Job drawing, mm, ordinate dimensions from the low corner. One solid piece. Round coordinates to 2 decimals unless told otherwise and drop trailing zeros. Write each loop counter-clockwise with the first axis right and the second up, starting at its lowest first coordinate (ties: lowest second). Pieces come first, ordered by that corner, then holes.
1) Saw through at A-A (z = 58). Write the cut outline in (x, y).
2) Saw through at C-C (x = 2.3). Write the cut outline in (y, z), plus the area to 3 significant figures.
3) Saw through at B-B (y = 88). Write the cut outline in (x, z).
4) Saw through at D-D (z = 7.5). Write the cut outline in (x, y).
5) Wall check: probe 1 along Y at (x, z) = (2.7, 7.5); probe 2 along Z at (x, y) = (3.35, 105); probe 3 along Y at (x, z) = (2, 58). Give the ranges that are in metal, low to high.
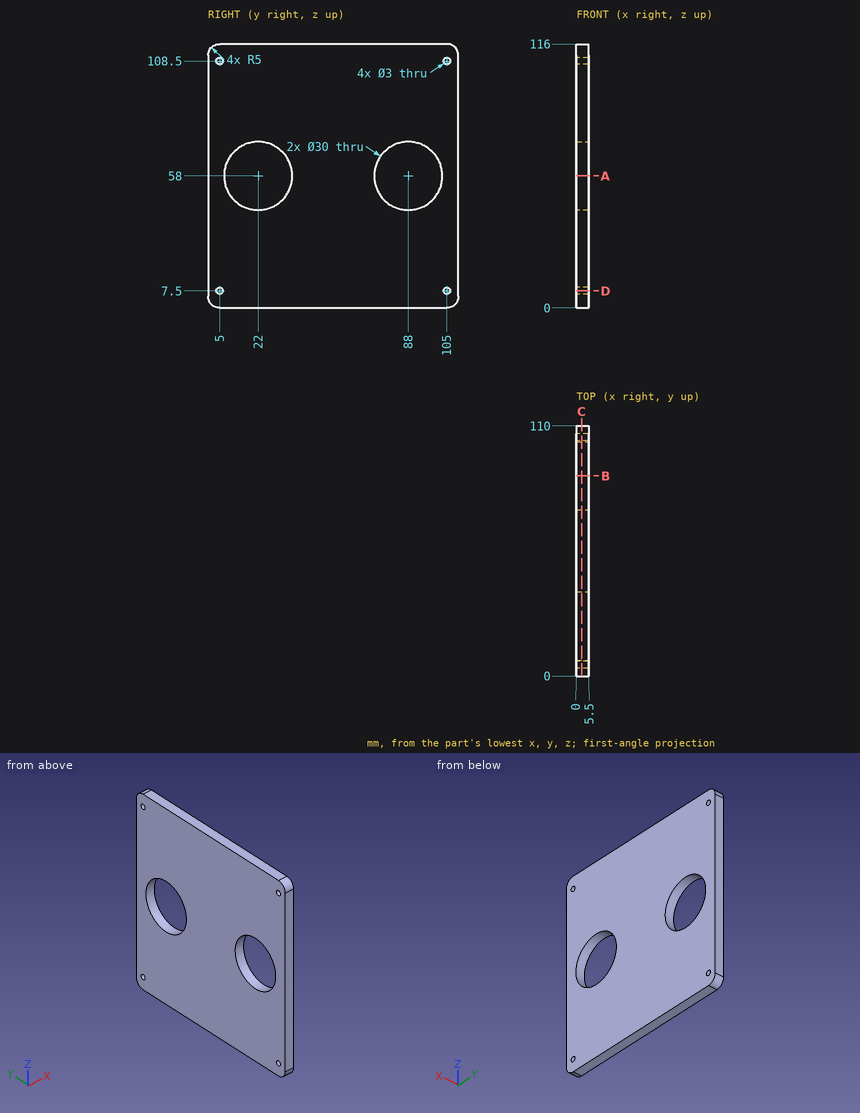
Evaluation:
1. outline: (0, 0) - (5.5, 0) - (5.5, 7) - (0, 7) - close; (0, 37) - (5.5, 37) - (5.5, 73) - (0, 73) - close; (0, 103) - (5.5, 103) - (5.5, 110) - (0, 110) - close
2. outline: (0, 5) arc R5 ccw to (5, 0) - (105, 0) arc R5 ccw to (110, 5) - (110, 111) arc R5 ccw to (105, 116) - (5, 116) arc R5 ccw to (0, 111) - close; hole circle Ø3 at (5, 7.5); hole circle Ø3 at (5, 108.5); hole circle Ø30 at (22, 58); hole circle Ø30 at (88, 58); hole circle Ø3 at (105, 7.5); hole circle Ø3 at (105, 108.5)
2. area: 11,300 mm2
3. outline: (0, 0) - (5.5, 0) - (5.5, 43) - (0, 43) - close; (0, 73) - (5.5, 73) - (5.5, 116) - (0, 116) - close
4. outline: (0, 0) - (5.5, 0) - (5.5, 3.5) - (0, 3.5) - close; (0, 6.5) - (5.5, 6.5) - (5.5, 103.5) - (0, 103.5) - close; (0, 106.5) - (5.5, 106.5) - (5.5, 110) - (0, 110) - close
5. probe 1: y = 0 to 3.5, 6.5 to 103.5, 106.5 to 110
5. probe 2: z = 0 to 6, 9 to 107, 110 to 116
5. probe 3: y = 0 to 7, 37 to 73, 103 to 110
